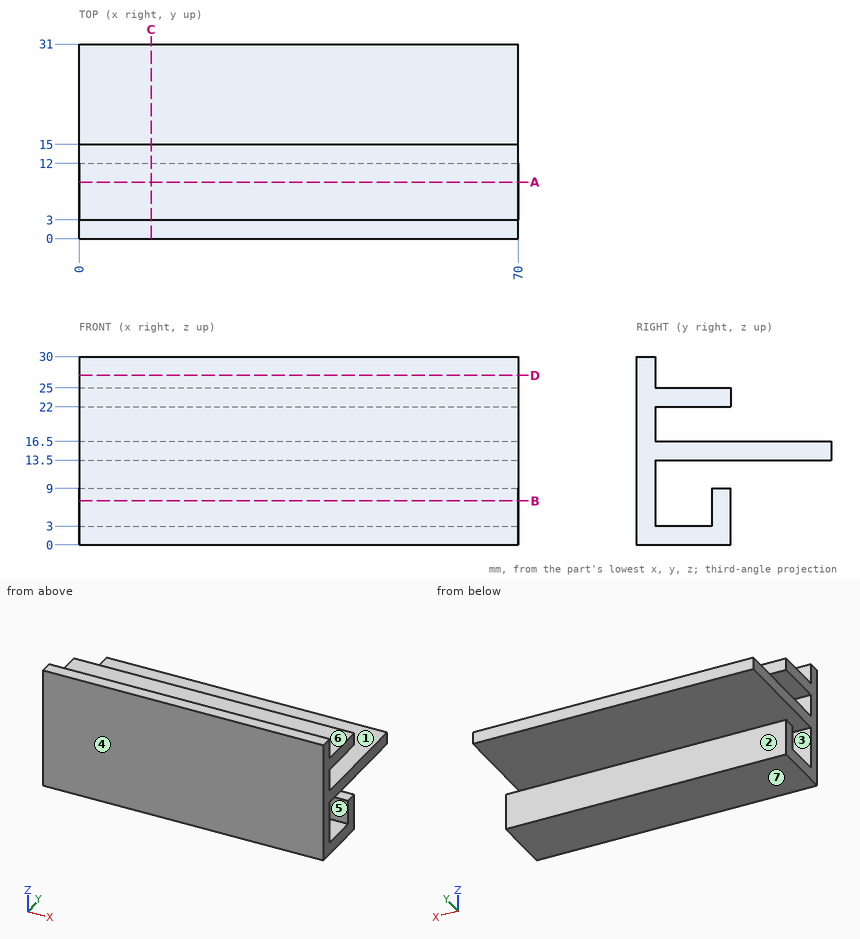
Here's the drawing with two shaded views (mm, measured from the low corner). I have some questions. A direction names the side the tool comes from. Coordinates: 2 decimals unless noted, no trailing zeros. Write each loop counter-clockwise with the first axis right and the second up, starting at its lowest first coordinate (ties: lowest second). Pieces come first, ordered by that corner, then holes.
Item 1: Will these pins go through, and if not, where does the flat tip stop? pin 1 (10 mm diameter, centred on x = 39, z = 6, fed in from +Y); pin 2 (1.5 mm diameter, centred on x = 26.5, y = 13, fed in from +Z); pin 3 (3 mm diameter, centred on y = 25, z = 19, fed in from +X); pin 4 (4 mm diameter, centred on x = 38.5, z = 27.5, fed in from +Y).
Item 2: If I drill on line 1 (Z direction, x = 53.5, y = 10); line 2 (Z direction, x = 7.5, y = 28.5); line 3 (Y direction, x = 20, z = 1.75), over which ranges is the centre line in solid material (lowest first)?
Item 3: I want a section at A-A on y = 9. Write out the boundary of the cut face in (x, z).
Item 4: I want a section at D-D on z = 27. Write out the boundary of the cut face in (x, y), and give its area (3 significant figures).
Item 5: I want a section at C-C on x = 11.5. Write out the boundary of the cut face in (y, z), and give its area (3 significant figures).
Item 6: If we mould it in two halves opening along Z, with no side actions, what happens to the marked faces 5, 6 and 7? For each: +Z half, -Z half, draft (parallel to the pull), parting line (faces both ways), or undercut.
Item 7: I want a section at B-B on z = 7. Write out the boundary of the cut face in (x, y), and give its area (3 significant figures).
Item 8: On a 3-axis mill with a long thin cutter (end or side, diameter ignored), from which of +Z, -Z, +X, -X, +Y, -Y can I reach the whole of each face in a straight line? I mean the marked faces 1, 2, 3 and 4. Say none if no direction works.
Findings below:
1. pin 1: stops at y = 15
1. pin 2: stops at z = 25
1. pin 3: passes through
1. pin 4: stops at y = 3
2. line 1: z = 0 to 3, 13.5 to 16.5, 22 to 25
2. line 2: z = 13.5 to 16.5
2. line 3: y = 0 to 15
3. outline: (0, 0) - (70, 0) - (70, 3) - (0, 3) - close; (0, 13.5) - (70, 13.5) - (70, 16.5) - (0, 16.5) - close; (0, 22) - (70, 22) - (70, 25) - (0, 25) - close
4. outline: (0, 0) - (70, 0) - (70, 3) - (0, 3) - close
4. area: 210 mm2
5. outline: (0, 0) - (15, 0) - (15, 9) - (12, 9) - (12, 3) - (3, 3) - (3, 13.5) - (31, 13.5) - (31, 16.5) - (3, 16.5) - (3, 22) - (15, 22) - (15, 25) - (3, 25) - (3, 30) - (0, 30) - close
5. area: 264 mm2
6. face 5: undercut
6. face 6: +Z half
6. face 7: -Z half
7. outline: (0, 0) - (70, 0) - (70, 3) - (0, 3) - close; (0, 12) - (70, 12) - (70, 15) - (0, 15) - close
7. area: 420 mm2
8. face 1: +X, -X, +Y
8. face 2: -Z, +X, -X, +Y
8. face 3: +X, -X
8. face 4: +Z, -Z, +X, -X, -Y
